Geometry check sheet. Reference: the model listing, model coordinates, mm. Round coordinates to 2 decimals unless told otherwise and drop trailing zeros. Order: outer loops, then holes, each group sorted by start corner. A loop starts at its lowest first (then second) coordinate and runs counter-clockwise, first axis right, second up.
(1) Cross-section at B-B on x = -44. Enter the section's corners in (y, z) (3 decimals).
(2) Thickness scan on L1, parallel to X at y = -2.4, z = 23.5; L2, parallel to Z at x = -23.5, y = -1.7 (3 decimals); L3, parallel to X at y = -1.05, z = 44. Record the ranges inside material, lowest first.
(3) Cross-section at D-D on x = -30. Enter the section's corners in (y, z) (3 decimals).
(4) Cross-section at C-C on y = -1.4. Count the separate pieces of the cut face and the enclosed holes in it, and give its area (3 significant figures).
(5) Cross-section at A-A on z = 0. Enter the section's corners in (x, y) (3 decimals), and give its area (3 significant figures).
(6) Gauge pin test, flat ends, axial feed: P1, Ø1, axis at y = -1.5, z = -30, coming from the -X side; P2, Ø8, axis at x = -23.5, z = -23.5, coming from the +Y side; P3, Ø23, axis at x = 0, z = 0, coming from the -Y side; P4, Ø1.5, axis at y = -1, z = 9.5, coming from the -X side. Record the tip position at first contact, or that the pin passes through.
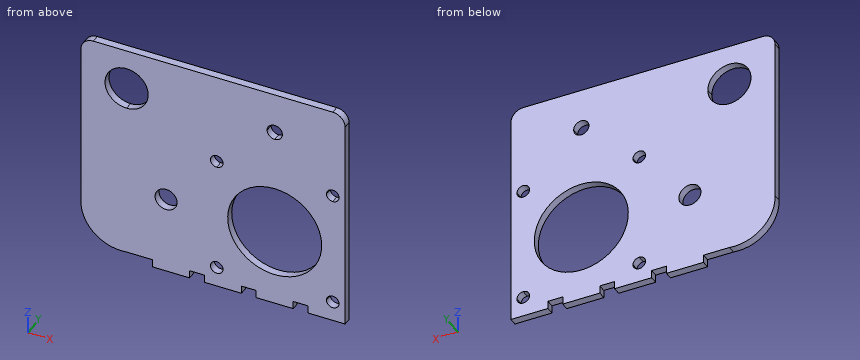
from build123d import *

# Parameters (mm, degrees)
F0_W     = 15
F0_H     = 3.175
F0_W_2   = 7.5
F0_R     = 4.4670073426
F1_DEPTH = 3.175


# Not quite as in the source:
# - a feature names something its author has since deleted; it is built from what else it names


with BuildPart() as f1:
    # F0 (on Front) → F1 (new body)
    with BuildSketch(Plane.XZ):
        with BuildLine():
            Line((0, 19.05), (0, 23.5))
            Line((0, 23.5), (-20.95, 23.5))
            ThreePointArc((-20.95, 23.5), (-21.696877708, 21.696877708), (-23.5, 20.95))
            Line((-23.5, 20.95), (-23.5, 0))
            Line((-23.5, 0), (-19.05, 0))
            ThreePointArc((-19.05, 0), (-13.4703841816, 13.4703841816), (0, 19.05))
        make_face()
        with BuildLine():
            Line((20.95, 23.5), (0, 23.5))
            Line((0, 23.5), (0, 19.05))
            ThreePointArc((0, 19.05), (13.4703841816, 13.4703841816), (19.05, 0))
            ThreePointArc((19.05, 0), (0, -19.05), (-19.05, 0))
            Line((-19.05, 0), (-23.5, 0))
            Line((-23.5, 0), (-23.5, -20.95))
            ThreePointArc((-23.5, -20.95), (-21.696877708, -21.696877708), (-20.95, -23.5))
            Line((-20.95, -23.5), (20.95, -23.5))
            ThreePointArc((20.95, -23.5), (21.696877708, -21.696877708), (23.5, -20.95))
            Line((23.5, -20.95), (23.5, 20.95))
            ThreePointArc((23.5, 20.95), (21.696877708, 21.696877708), (20.95, 23.5))
        make_face()
        with Locations((21, -30.0875)):
            Rectangle(F0_W, F0_H)
        with Locations((3.75, -30.0875)):
            Rectangle(F0_W_2, F0_H)
        with Locations((-3.75, -30.0875)):
            Rectangle(F0_W_2, F0_H)
        with Locations((-21, -30.0875)):
            Rectangle(F0_W, F0_H)
        with BuildLine():
            Line((0, 28.5), (-28.5, 28.5))
            Line((-28.5, 28.5), (-28.5, 0))
            Line((-28.5, 0), (-23.5, 0))
            Line((-23.5, 0), (-23.5, 20.95))
            ThreePointArc((-23.5, 20.95), (-25.303122292, 25.303122292), (-20.95, 23.5))
            Line((-20.95, 23.5), (0, 23.5))
            Line((0, 23.5), (0, 28.5))
        make_face()
        with BuildLine():
            Line((23.5, 28.5), (0, 28.5))
            Line((0, 28.5), (0, 23.5))
            Line((0, 23.5), (20.95, 23.5))
            ThreePointArc((20.95, 23.5), (23.5, 26.05), (26.05, 23.5))
            ThreePointArc((26.05, 23.5), (25.303122292, 21.696877708), (23.5, 20.95))
            Line((23.5, 20.95), (23.5, -20.95))
            ThreePointArc((23.5, -20.95), (25.303122292, -21.696877708), (26.05, -23.5))
            ThreePointArc((26.05, -23.5), (23.5, -26.05), (20.95, -23.5))
            Line((20.95, -23.5), (-20.95, -23.5))
            ThreePointArc((-20.95, -23.5), (-25.303122292, -25.303122292), (-23.5, -20.95))
            Line((-23.5, -20.95), (-23.5, 0))
            Line((-23.5, 0), (-28.5, 0))
            Line((-28.5, 0), (-28.5, -28.5))
            Line((-28.5, -28.5), (-13.5, -28.5))
            Line((-13.5, -28.5), (-7.5, -28.5))
            Line((-7.5, -28.5), (0, -28.5))
            Line((0, -28.5), (7.5, -28.5))
            Line((7.5, -28.5), (13.5, -28.5))
            Line((13.5, -28.5), (28.5, -28.5))
            Line((28.5, -28.5), (28.5, 23.5))
            Line((28.5, 23.5), (28.5, 28.5))
            Line((28.5, 28.5), (23.5, 28.5))
        make_face()
        with BuildLine():
            Line((-51.25, 44), (-28.5, 44))
            Line((-28.5, 44), (-28.5, 60.5991594493))
            Line((-28.5, 60.5991594493), (-73.5, 60.5991594493))
            ThreePointArc((-73.5, 60.5991594493), (-77.0355339059, 59.1346933553), (-78.5, 55.5991594493))
            Line((-78.5, 55.5991594493), (-78.5, -11.5))
            ThreePointArc((-78.5, -11.5), (-73.1911039749, -24.2888484433), (-60, -28.5))
            Line((-60, -28.5), (-60, 35.25))
            ThreePointArc((-60, 35.25), (-66.1871843354, 50.1871843354), (-51.25, 44))
        make_face()
        with BuildLine():
            Line((-28.5, 0), (-28.5, 28.5))
            Line((-28.5, 28.5), (-28.5, 44))
            Line((-28.5, 44), (-51.25, 44))
            ThreePointArc((-51.25, 44), (-53.8128156646, 37.8128156646), (-60, 35.25))
            Line((-60, 35.25), (-60, -28.5))
            Line((-60, -28.5), (-49.5, -28.5))
            Line((-49.5, -28.5), (-34.5, -28.5))
            Line((-34.5, -28.5), (-28.5, -28.5))
            Line((-28.5, -28.5), (-28.5, 0))
        make_face()
        with Locations((-44, 0)):
            Circle(F0_R, mode=Mode.SUBTRACT)
        with Locations((-42, -30.0875)):
            Rectangle(F0_W, F0_H)
        with BuildLine():
            Line((-28.5, 44), (-28.5, 28.5))
            Line((-28.5, 28.5), (0, 28.5))
            Line((0, 28.5), (0, 40.9))
            ThreePointArc((0, 40.9), (-2.1920310217, 41.8079689783), (-3.1, 44))
            Line((-3.1, 44), (-28.5, 44))
        make_face()
        with BuildLine():
            Line((0, 40.9), (0, 28.5))
            Line((0, 28.5), (23.5, 28.5))
            Line((23.5, 28.5), (28.5, 28.5))
            Line((28.5, 28.5), (28.5, 55.5991594493))
            ThreePointArc((28.5, 55.5991594493), (27.0355339059, 59.1346933553), (23.5, 60.5991594493))
            Line((23.5, 60.5991594493), (-28.5, 60.5991594493))
            Line((-28.5, 60.5991594493), (-28.5, 44))
            Line((-28.5, 44), (-3.1, 44))
            ThreePointArc((-3.1, 44), (0, 47.1), (3.1, 44))
            ThreePointArc((3.1, 44), (2.1920310217, 41.8079689783), (0, 40.9))
        make_face()
    extrude(amount=F1_DEPTH)


solid = f1.part
Found:
1. outline: (-3.175, -31.675) - (0, -31.675) - (0, -4.467) - (-3.175, -4.467) - close; (-3.175, 4.467) - (0, 4.467) - (0, 60.599) - (-3.175, 60.599) - close
2. L1: x = -78.5 to -26.05, -20.95 to 20.95, 26.05 to 28.5
2. L2: z = -31.675 to -26.05, -20.95 to 20.95, 26.05 to 60.599
2. L3: x = -78.5 to -68.75, -51.25 to -3.1, 3.1 to 28.5
3. outline: (-3.175, -28.5) - (0, -28.5) - (0, 60.599) - (-3.175, 60.599) - close
4. separate pieces: 1
4. enclosed holes: 8
4. area: 8,100 mm2
5. outline: (-78.5, -3.175) - (-48.467, -3.175) - (-48.467, 0) - (-78.5, 0) - close; (-39.533, -3.175) - (-19.05, -3.175) - (-19.05, 0) - (-39.533, 0) - close; (19.05, -3.175) - (28.5, -3.175) - (28.5, 0) - (19.05, 0) - close
5. area: 190 mm2
6. P1: stops at x = -49.5
6. P2: stops at y = 0
6. P3: passes through
6. P4: stops at x = -78.5
